Can you work these out from the model? Positions are in its coordinate system, mm. A direction names the side the tool comes from. Round coordinates to 2 decimals unless told otherwise and drop trailing zeros. Loops run counter-clockwise (first coordinate to the right, second up) from the corner with the lowest first, then second, coordinate; pieces in that order, holes last. Notation, with made-up numbers: M 66,29.25 L 88,29.25 A26 ccw 88,52.25 Z; hole C -40,2 d8. An arc over 180 degrees is marked long. Answer as CSV lines item,"result".
from build123d import *

# Parameters (mm, degrees)
EXTRUDE_1_DEPTH     = 10
SKETCH_2_R          = 7.5
CUT_EXTRUDE_1_DEPTH = 275.118587593
SKETCH_3_R          = 7.5
CUT_EXTRUDE_2_DEPTH = 275.118587593
CUT_EXTRUDE_3_DEPTH = 275.118587593


with BuildPart() as part:
    # 草图1 → 凸台-拉伸1 (new body)
    with BuildSketch(Plane(origin=(0, 0, 0), x_dir=(1, 0, 0), z_dir=(0, 1, 0))):
        with BuildLine():
            ThreePointArc((0, 0), (-20, -20), (0, -40))
            add(Edge.make_bspline(
                [(0, -40), (125.5, -30), (251, -40)],
                knots=[0, 0, 0, 1, 1, 1], degree=2))
            ThreePointArc((251, -40), (271, -20), (251, 0))
            add(Edge.make_bspline(
                [(0, 0), (125.5, -10), (251, 0)],
                knots=[0, 0, 0, 1, 1, 1], degree=2))
        make_face()
    extrude(amount=EXTRUDE_1_DEPTH)

    # 草图2 → 切除-拉伸1 (cut, through all)
    with BuildSketch(Plane(origin=(0, 10, 0), x_dir=(1, 0, 0), z_dir=(0, 1, 0))):
        with Locations(Location((0, -20, 0), (0, 0, 270))):
            Circle(SKETCH_2_R)
    extrude(amount=-CUT_EXTRUDE_1_DEPTH, mode=Mode.SUBTRACT)

    # 草图3 → 切除-拉伸2 (cut, through all)
    with BuildSketch(Plane(origin=(0, 10, 0), x_dir=(1, 0, 0), z_dir=(0, 1, 0))):
        with Locations(Location((251, -20, 0), (0, 0, 270))):
            Circle(SKETCH_3_R)
    extrude(amount=-CUT_EXTRUDE_2_DEPTH, mode=Mode.SUBTRACT)

    # 草图4 → 切除-拉伸3 (cut, through all)
    with BuildSketch(Plane(origin=(0, 10, 0), x_dir=(1, 0, 0), z_dir=(0, 1, 0))):
        Polygon((22.799917897, -11.455899991), (22.799917897, -27.860572008), (87.735077962, -19.658236), align=None)
        Polygon((229.567138104, -11.455899991), (229.567138104, -27.860572008), (170.98456159, -20.460667606), align=None)
    extrude(amount=-CUT_EXTRUDE_3_DEPTH, mode=Mode.SUBTRACT)


solid = part.part
Item 1: On a 3-axis mill with a long thin cutter (end or side, diameter ignored), from which of +Z, -Z, +X, -X, +Y, -Y can I reach the whole of each face in a straight line? I mean faces 4 (the face through (22.8, 5, 20)), 5 (the face through (123, 10, 20)). Say none if no direction works.
Output:
face 4,"+Y, -Y"
face 5,"+Z, -Z, +X, -X, +Y"
Item 2: Will these pins go through, and if not, where does the flat tip stop? pin 1 (3 mm diameter, centred on y = 3.5, z = 31.5, fed in from -X); pin 2 (4 mm diameter, centred on x = 122, y = 7.5, fed in from +Z); pin 3 (6 mm diameter, centred on y = 2.5, z = 32.5, fed in from +X).
Output:
pin 1,"stops at x = -17.32"
pin 2,"stops at z = 35.01"
pin 3,"stops at x = 268.6"
Item 3: If we section it at A-A on z = 23.5: Write out the boundary of the cut face in (x, y).
Output:
outline,"M -19.69,0 L -6.63,0 L -6.63,10 L -19.69,10 Z; M 6.63,0 L 22.8,0 L 22.8,10 L 6.63,10 Z; M 57.32,0 L 195.05,0 L 195.05,10 L 57.32,10 Z; M 229.57,0 L 244.37,0 L 244.37,10 L 229.57,10 Z; M 257.63,0 L 270.69,0 L 270.69,10 L 257.63,10 Z"
Item 4: We'd pull the mould along Z, two halves only. Please class faces 1 (the face through (271, 5, 20)), 2 (the face through (123, 0, 20)), 3 (the face through (229.567, 5, 20)): released by +Z, released by -Z, zero draft, split by the parting line, or undercut.
Output:
face 1,"split by the parting line"
face 2,"zero draft"
face 3,"undercut"
Item 5: If I drill on line 1 along Z through (x, y) = (122.5, 4); line 2 along Z through (x, y) = (64.5, 5.5); line 3 along Z through (x, y) = (215.5, 0.75), over which ranges is the centre line in solid material (lowest first)? Write a range as from..to.
Output:
line 1,"z = 5..35"
line 2,"z = 3.82..16.72, 22.59..36.18"
line 3,"z = 2.43..13.62, 26.08..37.57"
Item 6: If we section it at B-B on y = 2.25: State how many separate pieces and enclosed holes the cut face has, then the cut area to 3 significant figures.
Output:
separate pieces,"1"
enclosed holes,"4"
area,"8,260 mm2"
Item 7: If we section it at C-C on z = 9: Write out the boundary of the cut face in (x, y).
Output:
outline,"M -16.7,0 L 267.7,0 L 267.7,10 L -16.7,10 Z"
